```python
from build123d import *

# Parameters (mm, degrees)
F0_R     = 5
F1_DEPTH = 50
F2_R     = 1
F3_SIZE  = 1


with BuildPart() as f1:
    # F0 (on Top) → F1 (new body)
    with BuildSketch(Plane.XY):
        Circle(F0_R)
    extrude(amount=F1_DEPTH)

    # F2
    f2_edges = [f1.edges().sort_by_distance(p)[0] for p in [
        (-5, 0, 50),
    ]]
    fillet(f2_edges, radius=F2_R)

    # F3
    f3_edges = [f1.edges().sort_by_distance(p)[0] for p in [
        (-5, 0, 0),
    ]]
    chamfer(f3_edges, length=F3_SIZE)

    # F4: F1 across face


with BuildPart() as f1_1:
    add(f1.part)
    add(f1.part.mirror(Plane.XY.offset(50)))


solid = f1_1.part
```
Geometry check sheet. Reference: the model listing, model coordinates, mm. Round coordinates to 2 decimals unless told otherwise and drop trailing zeros. Write each loop counter-clockwise with the first axis right and the second up, starting at its lowest first coordinate (ties: lowest second). Pieces come first, ordered by that corner, then holes. Notation, with made-up numbers: (-2, -4.75) -> (5, -4.75) arc R8 ccw to (5, 3.25) -> close; hole circle Ø2 at (-30, 75.5). An arc over 180 degrees is marked (long way). Put each result on its own line as item: value.
1) Depth check by flat-ended pin: P1, Ø2, axis at y = -3.5, z = 34.5, coming from the -X side. Enter the tip coordinate at first touch or a pass-through.
Recorded:
P1: stops at x = -4.33
2) Cross-section at A-A, the plane z = 31. Enter the section's corners in (x, y), plus the area to 3 significant figures.
Recorded:
outline: circle Ø10 at (0, 0)
area: 78.5 mm2
3) Thickness scan on probe 1 along Z at (x, y) = (0.25, 4.5); probe 2 along X at (y, z) = (3, 25); probe 3 along Y at (x, z) = (0.25, 64.5). Record the ranges inside material, lowest first. Write a range as from..to.
Recorded:
probe 1: z = 0.51..49.86, 50.14..99.49
probe 2: x = -4..4
probe 3: y = -4.99..4.99
